Job drawing, mm, ordinate dimensions from the low corner. One solid piece. A direction names the side the tool comes from. Give positions to 0.01 mm unless a question says otherwise; leave off trailing zeros. Write each loop counter-clockwise with the first axis right and the second up, starting at its lowest first coordinate (ties: lowest second). Pieces come first, ordered by that corner, then holes. Notation, with made-up numbers: (62.5, 80.25) - (109.5, 80.25) arc R35 ccw to (109.5, 119.25) - close; hole circle Ø2 at (87.5, -16.75). An arc over 180 degrees is marked (long way). Put each result on its own line as item: value. Start each with the question number.
1. Cut at B-B on z = 35. List the corners of the cut face in (x, y) (1 decimal), and give its area (3 significant figures).
2. Wall check: line 1 (Z direction, x = 22, y = 23); line 2 (Y direction, x = 17, z = 40) (1 decimal); line 3 (Y direction, x = 38, z = 25.5) (1 decimal). Give the ranges that are in metal, low to high.
3. Mould opens along Z. For the marked faces 1, 2, 3 and 4 say: +Z half, -Z half, draft (parallel to the pull), parting line (faces both ways), or undercut.
4. Tool access for the marked faces 5, 6, 7, 8 and 9: list every direction of +Z, -Z, +X, -X, +Y, -Y with a clear straight run to the whole face (end or side of a thin tool).
5. Drop flat-ended pins along their axis: pin 1 (6.5 mm diameter, centred on y = 4, z = 13.5, fed in from -X); pin 2 (8 mm diameter, centred on x = 9, z = 11, fed in from +Y); pin 3 (5 mm diameter, centred on x = 12.5, y = 33, fed in from -Z). Give the stop position or say it passes through.
6. Cut at C-C on y = 32.5. List the corners of the cut face in (x, z).
7. Cut at D-D on x = 5. List the corners of the cut face in (y, z) (1 decimal).
8. Cut at A-A on x = 13.5. List the corners of the cut face in (y, z) (1 decimal).
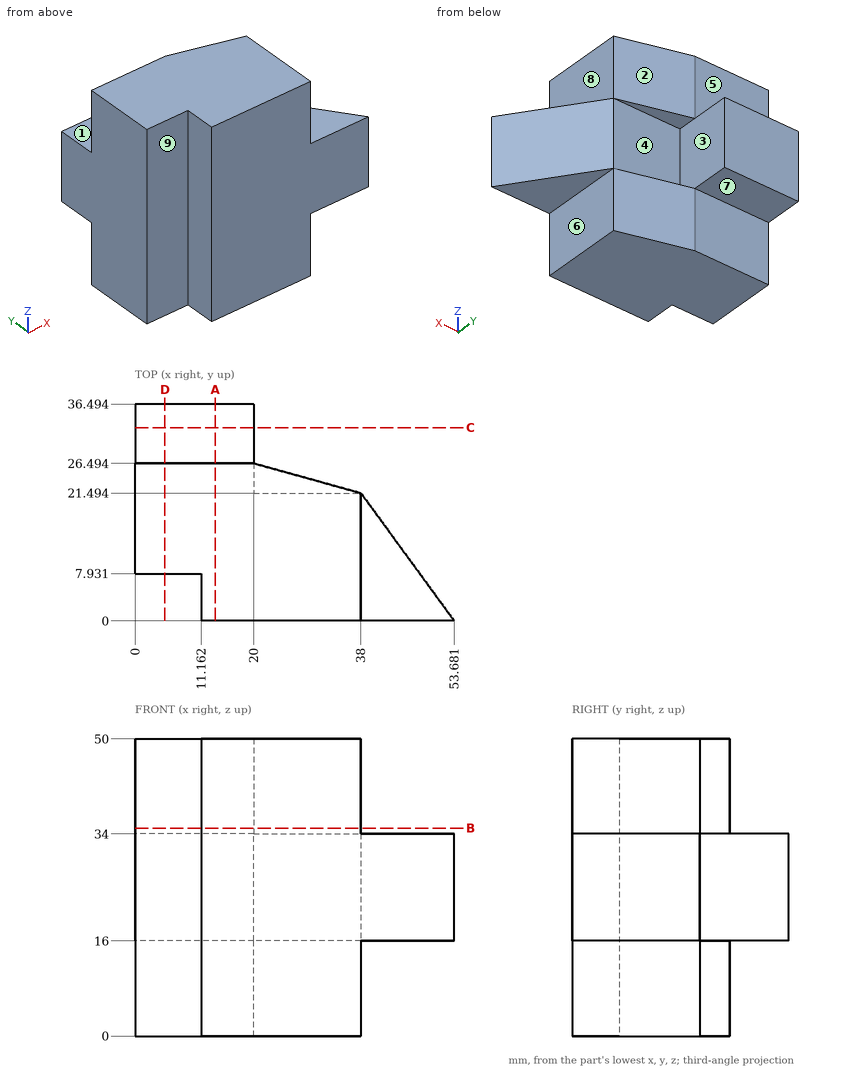
Report:
1. outline: (0, 7.9) - (11.2, 7.9) - (11.2, 0) - (38, 0) - (38, 21.5) - (20, 26.5) - (0, 26.5) - close
1. area: 873 mm²
2. line 1: z = 0 to 16, 34 to 50
2. line 2: y = 0 to 26.5
2. line 3: y = 0 to 21.5
3. face 1: +Z half
3. face 2: draft
3. face 3: undercut
3. face 4: undercut
4. face 5: +Z, +X, -X, +Y
4. face 6: -Z, +X, +Y, -Y
4. face 7: -Z, +X, -X, +Y
4. face 8: +Z, +X, +Y, -Y
4. face 9: +Z, -Z, -X, -Y
5. pin 1: stops at x = 11.16
5. pin 2: stops at y = 26.49
5. pin 3: stops at z = 16
6. outline: (0, 16) - (20, 16) - (20, 34) - (0, 34) - close
7. outline: (7.9, 0) - (26.5, 0) - (26.5, 16) - (36.5, 16) - (36.5, 34) - (26.5, 34) - (26.5, 50) - (7.9, 50) - close
8. outline: (0, 0) - (26.5, 0) - (26.5, 16) - (36.5, 16) - (36.5, 34) - (26.5, 34) - (26.5, 50) - (0, 50) - close
